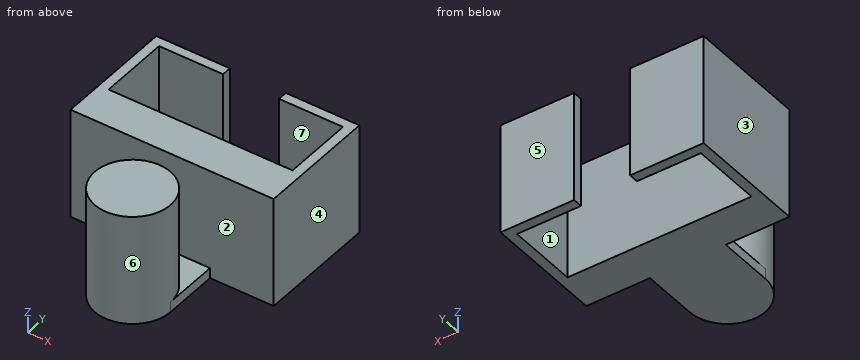
```python
from build123d import *

# Parameters (mm, degrees)
SKETCH1_R           = 13.081
BOSS_EXTRUDE1_DEPTH = 38.1
SKETCH2_W           = 26.162
SKETCH2_H           = 19.05
BOSS_EXTRUDE2_DEPTH = 3.556
SKETCH4_W           = 63.5
SKETCH4_H           = 38.1
BOSS_EXTRUDE3_DEPTH = 13.716
SKETCH6_W           = 38.1
SKETCH6_H           = 38.1
BOSS_EXTRUDE4_DEPTH = 3.302
SKETCH7_W           = 25.4
SKETCH7_H           = 38.1
BOSS_EXTRUDE5_DEPTH = 3.302


with BuildPart() as part:
    # Sketch1 → Boss-Extrude1 (new body)
    with BuildSketch(Plane.XY):
        with Locations(Location((0, 0, 0), (0, 0, 180))):
            Circle(SKETCH1_R)
    extrude(amount=BOSS_EXTRUDE1_DEPTH)

    # Sketch2 → Boss-Extrude2 (add)
    with BuildSketch(Plane(origin=(0, 0, 0), x_dir=(-1, 0, 0), z_dir=(0, 0, -1))):
        with Locations((0, 9.525)):
            Rectangle(SKETCH2_W, SKETCH2_H)
    extrude(amount=-BOSS_EXTRUDE2_DEPTH)

    # Sketch4 → Boss-Extrude3 (add)
    with BuildSketch(Plane(origin=(0, 19.05, 0), x_dir=(1, 0, 0), z_dir=(0, 1, 0))):
        with Locations((0, -19.05)):
            Rectangle(SKETCH4_W, SKETCH4_H)
    extrude(amount=BOSS_EXTRUDE3_DEPTH)

    # Sketch6 → Boss-Extrude4 (add)
    with BuildSketch(Plane(origin=(31.75, 0, 0), x_dir=(0, 0, -1), z_dir=(1, 0, 0))):
        with Locations((-19.05, 38.1)):
            Rectangle(SKETCH6_W, SKETCH6_H)
    boss_extrude4 = extrude(amount=BOSS_EXTRUDE4_DEPTH)

    # Mirror1: Boss-Extrude4 across plane
    add(boss_extrude4.mirror(Plane(origin=(0, 0, 0), x_dir=(0, 0, 1), z_dir=(1, 0, 0))))

    # Sketch7 → Boss-Extrude5 (add)
    with BuildSketch(Plane(origin=(0, 57.15, 0), x_dir=(1, 0, 0), z_dir=(0, 1, 0))):
        with Locations((22.352, -19.05)):
            Rectangle(SKETCH7_W, SKETCH7_H)
    boss_extrude5 = extrude(amount=BOSS_EXTRUDE5_DEPTH)

    # Mirror2: Boss-Extrude5 across plane
    add(boss_extrude5.mirror(Plane(origin=(0, 0, 0), x_dir=(0, 0, 1), z_dir=(1, 0, 0))))


solid = part.part
```
Model file for the job. Use its own axes, mm. Face numbers are marked on the shaded views. A direction names the side the tool comes from. Give positions to 0.01 mm unless a question says otherwise; leave off trailing zeros. Loops run counter-clockwise (first coordinate to the right, second up) from the corner with the lowest first, then second, coordinate; pieces in that order, holes last. Notation, with made-up numbers: (64.5, 83.25) -> (99.5, 83.25) arc R12 ccw to (99.5, 101.25) -> close; hole circle Ø1 at (76, 61.25). An arc over 180 degrees is marked (long way). Use CSV: the item, a comma, the result in double quotes. Start each with the question number.
1) Slice it at D-D on y = 18. Give the cut face in (x, z), plus the area to 3 significant figures.
2) Slice it at C-C on x = 0. Give the cut face in (y, z), plus the area to 3 significant figures.
3) Flat gauge pins, fed straight in: pin 1 Ø6.5 at (x, z) = (16.5, 15.5) entering from -Y; pin 2 Ø1.8 at (y, z) = (10.5, 2) entering from +X; pin 3 Ø4 at (x, z) = (13.5, 25) entering from -Y. Where does each tip first touch, or does it go through?
4) Wall check: line 1 (X direction, y = 47.5, z = 29); line 2 (Y direction, x = 24, z = 8.5); line 3 (Y direction, x = -10.5, z = 6). Give the ranges that are in metal, low to high.
5) Slice it at A-A on z = 18.5. Give the cut face in (x, y).
6) Mould opens along X. For the marked faces 1, 2, 3 and 4 say: released by +X, released by -X, zero draft, split by the parting line, or undercut.
7) Tool access for the marked faces 5, 6 and 7: list every direction of +Z, -Z, +X, -X, +Y, -Y with a clear straight run to the whole face (end or side of a thin tool).
8) Slice it at B-B on x = 26. Give the cut face in (y, z).
Computed values:
1,outline,"(-13.08, 0) -> (13.08, 0) -> (13.08, 3.56) -> (-13.08, 3.56) -> close"
1,area,"93.0 mm^2"
2,outline,"(-13.08, 0) -> (32.77, 0) -> (32.77, 38.1) -> (19.05, 38.1) -> (19.05, 3.56) -> (13.08, 3.56) -> (13.08, 38.1) -> (-13.08, 38.1) -> close"
2,area,"1,540 mm^2"
3,pin 1,"stops at y = 19.05"
3,pin 2,"stops at x = 13.08"
3,pin 3,"stops at y = -6.23"
4,line 1,"x = -35.05 to -31.75, 31.75 to 35.05"
4,line 2,"y = 19.05 to 32.77, 57.15 to 60.45"
4,line 3,"y = -7.8 to 7.8, 19.05 to 32.77, 57.15 to 60.45"
5,outline,"(-35.05, 19.05) -> (35.05, 19.05) -> (35.05, 60.45) -> (9.65, 60.45) -> (9.65, 57.15) -> (31.75, 57.15) -> (31.75, 32.77) -> (-31.75, 32.77) -> (-31.75, 57.15) -> (-9.65, 57.15) -> (-9.65, 60.45) -> (-35.05, 60.45) -> close; circle Ø26.16 at (0, 0)"
6,face 1,"undercut"
6,face 2,"zero draft"
6,face 3,"released by -X"
6,face 4,"released by +X"
7,face 5,"+Z, -Z, +X, -X, +Y"
7,face 6,"+Z"
7,face 7,"+Z, -Z"
8,outline,"(19.05, 0) -> (32.77, 0) -> (32.77, 38.1) -> (19.05, 38.1) -> close; (57.15, 0) -> (60.45, 0) -> (60.45, 38.1) -> (57.15, 38.1) -> close"
